Could you check a few things on this model? Use its own coordinates, in mm. A direction names the side the tool comes from. Give positions to 0.01 mm unless a question says otherwise; leave off trailing zeros. Loops run counter-clockwise (first coordinate to the right, second up) from the corner with the lowest first, then second, coordinate; pieces in that order, holes last. Notation, with made-up numbers: M -21.5,65 L 26.5,65 A14 cw 26.5,75 Z; hole C 77,-33.75 d7. An arc over 180 degrees is marked long. Use a Markdown table: item, result. Add a question column.
1) We'd pull the mould along Z, two halves only. Please class faces 1 (the flat face through (-47.527, -174.326, -44.033)), 2 (the flat face through (1.7, -2.5, 46.72)), 3 (the cylindrical face through (14.87, -88.49, 20.59)): +Z half, -Z half, draft (parallel to the pull), parting line (faces both ways), or undercut.
2) Suppose I cut it at B-B on z = 16.5. List the corners of the cut face in (x, y) for me, and give its area (3 significant figures).
3) If I drill on line 1 along Y through (x, z) = (-113, -11); line 2 along X through (y, z) = (-168, -96); line 3 along Z through (x, y) = (-47.5, -138), over which ranges is the centre line in solid material (lowest first)? Write a range as [from, to].
4) Which directions (+Z, -Z, +X, -X, +Y, -Y) give clear straight access to the entire face, cutting with the end or side of a thin tool? Please do faces 4 (the flat face through (-69, -172.72, -60)), 5 (the flat face through (43, -88, -47.173)), 6 (the flat face through (-69, -5.08, -60)).
5) Suppose I cut it at C-C on z = -29. List the corners of the cut face in (x, y) for me, and give its area (3 significant figures).
6) Will these pins go through, and if not, where does the flat tip stop? pin 1 Ø5 at (x, y) = (-0.5, -152) entering from -Z; pin 2 Ø6 at (y, z) = (-18, -83) entering from +X; pin 3 Ø4 at (x, z) = (-113.5, 14) entering from +Y.
7) Suppose I cut it at A-A on y = -112.5. List the corners of the cut face in (x, z) for me.
8) Suppose I cut it at D-D on x = 0. List the corners of the cut face in (y, z) for me, and give its area (3 significant figures).
```python
from build123d import *

# Parameters (mm, degrees)
F3_W       = 106.9038137794
F3_H       = 96.4715331793
F4_DEPTH   = 177.8
F5_SIZE    = 5.08
F1_D       = 50.8
F4_FACE1_W = 167.64
F4_FACE1_H = 86.3115331793


with BuildPart() as f4:
    # F3 (on Front) → F4 (new body)
    with BuildSketch(Plane.XZ):
        with Locations((2.3797191679, 1.0631904006)):
            Rectangle(F3_W, F3_H)
    extrude(amount=F4_DEPTH)

    # F5
    f5_edges = [f4.edges().sort_by_distance(p)[0] for p in [
        (55.831626, -88.9, 49.298957),
        (2.379719, -177.8, 49.298957),
        (-51.072188, -177.8, 1.06319),
        (2.379719, -177.8, -47.172576),
        (55.831626, -177.8, 1.06319),
        (2.379719, 0, 49.298957),
        (-51.072188, 0, 1.06319),
        (2.379719, 0, -47.172576),
        (55.831626, 0, 1.06319),
        (-51.072188, -88.9, -47.172576),
        (-51.072188, -88.9, 49.298957),
        (55.831626, -88.9, -47.172576),
    ]]
    chamfer(f5_edges, length=F5_SIZE)

    # F1 (through all)
    with Locations(Plane.XZ.offset(177.8)):
        with Locations((0, 0)):
            Hole(F1_D / 2)

    # F4_face1 (on face) → F2 (revolve)
    with BuildSketch(Plane(origin=(-51.0721877217, -88.9, 1.0631904006), x_dir=(0, -1, 0), z_dir=(-1, 0, 0))):
        Rectangle(F4_FACE1_W, F4_FACE1_H)
    revolve(axis=Axis((-51.0721877217, -88.9, -42.092576189), (0, 1, 0)))


solid = f4.part
```
Answer block:
| question | item | result |
|---|---|---|
| 1 | face 1 | -Z half |
| 1 | face 2 | +Z half |
| 1 | face 3 | undercut |
| 2 | outline | M -114.45,-172.72 L -51.07,-172.72 L -45.99,-177.8 L -19.31,-177.8 L -19.31,-172.72 L 12.3,-172.72 L 12.3,-5.08 L -19.31,-5.08 L -19.31,0 L -45.99,0 L -51.07,-5.08 L -114.45,-5.08 Z; M 19.31,-177.8 L 50.75,-177.8 L 55.83,-172.72 L 55.83,-5.08 L 50.75,0 L 19.31,0 Z |
| 2 | area | 28,000 mm^2 |
| 3 | line 1 | y = [-172.72, -5.08] |
| 3 | line 2 | x = [-118.48, 16.33] |
| 3 | line 3 | z = [-128.33, 47.79] |
| 4 | face 4 | -Z, -X, -Y |
| 4 | face 5 | -Z, +X, +Y, -Y |
| 4 | face 6 | -Z, -X, +Y |
| 5 | outline | M -136.38,-172.72 L -51.07,-172.72 L -45.99,-177.8 L 50.75,-177.8 L 55.83,-172.72 L 55.83,-5.08 L 50.75,0 L -45.99,0 L -51.07,-5.08 L -136.38,-5.08 Z |
| 5 | area | 33,300 mm^2 |
| 6 | pin 1 | stops at z = -113.78 |
| 6 | pin 2 | stops at x = 26.47 |
| 6 | pin 3 | stops at y = -5.08 |
| 7 | outline | M -51.07,44.22 A86.31 ccw long 35.09,-47.17 L 50.75,-47.17 L 55.83,-42.09 L 55.83,44.22 L 50.75,49.3 L -45.99,49.3 Z; hole M 2.94,25.23 A86.31 cw 25.33,-1.93 A25.4 ccw Z |
| 8 | outline | M -177.8,-42.09 L -172.72,-47.17 L -172.72,-111.67 L -5.08,-111.67 L -5.08,-47.17 L 0,-42.09 L 0,-25.4 L -5.08,-25.4 L -5.08,25.4 L 0,25.4 L 0,44.22 L -5.08,49.3 L -172.72,49.3 L -177.8,44.22 L -177.8,25.4 L -172.72,25.4 L -172.72,-25.4 L -177.8,-25.4 Z |
| 8 | area | 27,400 mm^2 |
